Design review of the part built by this model. Coordinates are the model's own, in mm. A direction names the side the tool comes from. Round coordinates to 2 decimals unless told otherwise and drop trailing zeros. Write each loop counter-clockwise with the first axis right and the second up, starting at its lowest first coordinate (ties: lowest second). Pieces come first, ordered by that corner, then holes.
from build123d import *

# Parameters (mm, degrees)
F1_DEPTH      = 254
F1_DEPTH_BACK = 254
F4_DEPTH      = 12.7
F6_D          = 6.35
F8_D          = 6.35
F8_DEPTH      = 12.7
F8_TIP        = 1.9077324654
F10_D         = 6.35
F12_D         = 6.35
F14_DEPTH     = 25.4
F15_R         = 5.08
F17_DEPTH     = 63.5
F19_D         = 6.35
F19_DEPTH     = 12.7
F19_TIP       = 1.9077324654


# Not quite as in the source:
# - a pattern or mirror of a feature is missing from the dataset's text; its kind, count and spacing are read off the source's solid
# - a feature names something its author has since deleted; it is built from what else it names


with BuildPart() as f1:
    # F0 (on Top) → F1 (new body, two sides)
    with BuildSketch(Plane.XY) as f1_sk:
        with BuildLine():
            Line((-50.8, -63.5), (50.8, -63.5))
            ThreePointArc((50.8, -63.5), (59.7802561211, -59.7802561211), (63.5, -50.8))
            Line((63.5, -50.8), (63.5, 50.8))
            ThreePointArc((63.5, 50.8), (59.7802561211, 59.7802561211), (50.8, 63.5))
            Line((50.8, 63.5), (-50.8, 63.5))
            ThreePointArc((-50.8, 63.5), (-59.7802561211, 59.7802561211), (-63.5, 50.8))
            Line((-63.5, 50.8), (-63.5, -50.8))
            ThreePointArc((-63.5, -50.8), (-59.7802561211, -59.7802561211), (-50.8, -63.5))
        make_face()
        with BuildLine():
            ThreePointArc((50.8, 57.1499988437), (55.2901272429, 55.2901272429), (57.1499988437, 50.8))
            Line((57.1499988437, 50.8), (57.1499988437, -50.8))
            ThreePointArc((57.1499988437, -50.8), (55.2901272429, -55.2901272429), (50.8, -57.1499988437))
            Line((50.8, -57.1499988437), (-50.8, -57.1499988437))
            ThreePointArc((-50.8, -57.1499988437), (-55.2901272429, -55.2901272429), (-57.1499988437, -50.8))
            Line((-57.1499988437, -50.8), (-57.1499988437, 50.8))
            ThreePointArc((-57.1499988437, 50.8), (-55.2901272429, 55.2901272429), (-50.8, 57.1499988437))
            Line((-50.8, 57.1499988437), (50.8, 57.1499988437))
        make_face(mode=Mode.SUBTRACT)
    extrude(amount=F1_DEPTH)
    extrude(f1_sk.sketch, amount=-F1_DEPTH_BACK)

    # F3 (on face) → F4 (join)
    with BuildSketch(Plane.XY.offset(254)):
        with BuildLine():
            Line((50.8, 57.1499988437), (25.4, 57.1499988437))
            Line((25.4, 57.1499988437), (25.4, -57.1499988437))
            Line((25.4, -57.1499988437), (50.8, -57.1499988437))
            ThreePointArc((50.8, -57.1499988437), (55.2901272429, -55.2901272429), (57.1499988437, -50.8))
            Line((57.1499988437, -50.8), (57.1499988437, 50.8))
            ThreePointArc((57.1499988437, 50.8), (55.2901272429, 55.2901272429), (50.8, 57.1499988437))
        make_face()
        with BuildLine():
            Line((-25.4, -57.1499988437), (-25.4, 57.1499988437))
            Line((-25.4, 57.1499988437), (-50.8, 57.1499988437))
            ThreePointArc((-50.8, 57.1499988437), (-55.2901272429, 55.2901272429), (-57.1499988437, 50.8))
            Line((-57.1499988437, 50.8), (-57.1499988437, -50.8))
            ThreePointArc((-57.1499988437, -50.8), (-55.2901272429, -55.2901272429), (-50.8, -57.1499988437))
            Line((-50.8, -57.1499988437), (-25.4, -57.1499988437))
        make_face()
    extrude(amount=-F4_DEPTH)

    # F6 (through all)
    with Locations(Plane.YZ.offset(63.5)):
        with Locations((0, 209.55), (0, 228.6)):
            Hole(F6_D / 2)

    # F8
    with Locations(Plane.XZ.offset(63.5)):
        with Locations((0, -228.6)):
            Hole(F8_D / 2, depth=F8_DEPTH)
            with Locations((0, 0, -(F8_DEPTH + F8_TIP / 2))):  # 118° drill point
                Cone(0, F8_D / 2, F8_TIP, mode=Mode.SUBTRACT)

    # F10 (through all)
    with Locations(Plane.YZ.offset(63.5)):
        with Locations((0, 0), (0, -127), (0, 127)):
            Hole(F10_D / 2)

    # F12 (through all)
    with Locations(Plane(origin=(0, 63.5, 0), x_dir=(-1, 0, 0), z_dir=(0, 1, 0))):
        with Locations((0, 0), (0, -127), (0, 127)):
            Hole(F12_D / 2)

    # F13 (on face) → F14 (cut)
    with BuildSketch(Plane(origin=(0, 63.5, 0), x_dir=(-1, 0, 0), z_dir=(0, 1, 0))):
        with BuildLine():
            Line((25.4, 196.85), (25.4, 254))
            Line((25.4, 254), (-25.4, 254))
            Line((-25.4, 254), (-25.4, 196.85))
            ThreePointArc((-25.4, 196.85), (-23.5401280605, 192.3598719395), (-19.05, 190.5))
            Line((-19.05, 190.5), (19.05, 190.5))
            ThreePointArc((19.05, 190.5), (23.5401280605, 192.3598719395), (25.4, 196.85))
        make_face()
    extrude(amount=-F14_DEPTH, mode=Mode.SUBTRACT)

    # F15
    f15_edges = [f1.edges().sort_by_distance(p)[0] for p in [
        (25.4, 63.5, 225.425),
        (-25.4, 3.175001, 254),
        (25.4, 3.175001, 254),
        (0, -57.149999, 254),
        (-25.4, 63.5, 225.425),
        (-23.540128, 63.5, 192.359872),
        (0, 63.5, 190.5),
        (23.540128, 63.5, 192.359872),
    ]]
    fillet(f15_edges, radius=F15_R)

    # F16 (on face) → F17 (join)
    with BuildSketch(Plane.XY.offset(254)):
        with BuildLine():
            Line((-63.5, 50.8), (-63.5, 41.8197438789))
            Line((-63.5, 41.8197438789), (-41.8197438789, 63.5))
            Line((-41.8197438789, 63.5), (-50.8, 63.5))
            ThreePointArc((-50.8, 63.5), (-59.7802561211, 59.7802561211), (-63.5, 50.8))
        make_face()
        with BuildLine():
            Line((-63.5, 63.5), (-63.5, 50.8))
            ThreePointArc((-63.5, 50.8), (-59.7802561211, 59.7802561211), (-50.8, 63.5))
            Line((-50.8, 63.5), (-63.5, 63.5))
        make_face()
    f17 = extrude(amount=-F17_DEPTH)

    # F17_copies: F17 across plane
    add(f17.mirror(Plane(origin=(0, 0, 0), x_dir=(0, 0, 1), z_dir=(1, 0, 0))))

    # F19
    with Locations(Plane(origin=(-63.5, 0, 0), x_dir=(0, -1, 0), z_dir=(-1, 0, 0))):
        with Locations((-48.26, 209.7200926909), (-50.8, 228.6)):
            f19 = Hole(F19_D / 2, depth=F19_DEPTH)
            with Locations((0, 0, -(F19_DEPTH + F19_TIP / 2))):  # 118° drill point
                Cone(0, F19_D / 2, F19_TIP, mode=Mode.SUBTRACT)

    # F19_copies: F19 across plane
    add(f19.mirror(Plane(origin=(-1e-06, 0, 0), x_dir=(0, 0, 1), z_dir=(1, 0, 0))), mode=Mode.SUBTRACT)


solid = f1.part
1) Add section A-A on z = 178.5. State the section outline as (x, y) points.
2) For line 1 along Y through (x, z) = (-61.75, 209.55) (3 decimals); line 2 along Z through (x, y) = (0, 59.25) (3 decimals); line 3 along Z through (x, y) = (-58, 0) (3 decimals), list the stretches that pass through material, from the lowest coordinate up.
3) The part is to be moulded in two halves that separate along X. For faces 1 (the face through (-59.88, -59.68, 3.56)), 2 (the face through (-57.15, 11, -3)), 3 (the face through (59.68, -59.88, 3.56)), say which applies: pulls with the +X half, pulls with the -X half, needs draft (parallel to the pull), parting line crosses it, or undercut.
4) Add section B-B on y = 38.5. State the section outline as (x, z) points, and give its area (3 significant figures).
5) For faces 4 (the face through (-5, -61, -254)), 5 (the face through (61, 60, 190.5)), 6 (the face through (11, 57.15, -3)), 7 (the face through (-59.68, 59.88, -28.64)), list the 3-axis set-ups (+Z, -Z, +X, -X, +Y, -Y) from which the entire face can be reached by the end or side of a thin tool; tool diameter is ignored.
6) For P1, Ø1, axis at x = 26, y = 2, coming from the +Z side; P2, Ø5, axis at x = 0, z = 0, coming from the +Y side; P3, Ø4.5, axis at x = 53, y = 53, coming from the -Z side, all flat-tipped, find the tip position at first contact; note any pin that passes through.
7) Add section C-C on x = 39.5. State the section outline as (y, z) points, and give its area (3 significant figures).
Computed:
1. outline: (-63.5, -50.8) arc R12.7 ccw to (-50.8, -63.5) - (50.8, -63.5) arc R12.7 ccw to (63.5, -50.8) - (63.5, 50.8) arc R12.7 ccw to (50.8, 63.5) - (-50.8, 63.5) arc R12.7 ccw to (-63.5, 50.8) - close; hole (-57.15, -50.8) arc R6.35 ccw to (-50.8, -57.15) - (50.8, -57.15) arc R6.35 ccw to (57.15, -50.8) - (57.15, 50.8) arc R6.35 ccw to (50.8, 57.15) - (-50.8, 57.15) arc R6.35 ccw to (-57.15, 50.8) - close
2. line 1: y = -57.233 to -3.175, 3.175 to 45.09, 51.43 to 63.5
2. line 2: z = -254 to -130.175, -123.825 to -3.175, 3.175 to 123.825, 130.175 to 190.432
2. line 3: z = -254 to -130.175, -123.825 to -3.175, 3.175 to 123.825, 130.175 to 206.375, 212.725 to 225.425, 231.775 to 254
3. face 1: pulls with the -X half
3. face 2: undercut
3. face 3: pulls with the +X half
4. outline: (-63.5, -254) - (-57.15, -254) - (-57.15, 241.3) - (-25.4, 241.3) - (-25.4, 248.92) arc R5.08 ccw to (-30.48, 254) - (-63.5, 254) - close; (25.4, 241.3) - (57.15, 241.3) - (57.15, -254) - (63.5, -254) - (63.5, 254) - (30.48, 254) arc R5.08 ccw to (25.4, 248.92) - close
4. area: 7,250 mm2
5. face 4: -Z, +X, -X, +Y, -Y
5. face 5: -Z, +X, +Y
5. face 6: -Z
5. face 7: -Z, -X, +Y
6. P1: stops at z = 252.08
6. P2: passes through
6. P3: stops at z = 190.5
7. outline: (-63.5, -254) - (-57.15, -254) - (-57.15, 241.3) - (57.15, 241.3) - (57.15, -254) - (63.5, -254) - (63.5, 254) - (-63.5, 254) - close
7. area: 7,900 mm2
